from build123d import *

# Parameters (mm, degrees)
F0_R         = 5
F0_R_2       = 1.75
F1_DEPTH     = 5.5
F3_DEPTH     = 3
F4_T4_DEPTH  = 14.8989794856
F4_S5_R      = 5
F4_T6_DEPTH  = 9
F4_T10_DEPTH = 14.8989794856
F4_S11_R     = 5
F4_T12_DEPTH = 9
F5_SIZE      = 0.5


# Not quite as in the source:
# - a fillet or chamfer that OpenCascade refuses, or shapes differently, is made with other operations: its cross-section is extruded or revolved along the edge and cut away or added


with BuildPart() as f1:
    # F0 (on Top) → F1 (new body)
    with BuildSketch(Plane.XY):
        Circle(F0_R)
        Circle(F0_R_2, mode=Mode.SUBTRACT)
    extrude(amount=F1_DEPTH)

    # F2 (on Top) → F3 (join)
    with BuildSketch(Plane.XY):
        with BuildLine():
            Line((0, -5), (4.8989794856, -5))
            ThreePointArc((4.8989794856, -5), (7, 0), (4.8989794856, 5))
            Line((4.8989794856, 5), (0, 5))
            ThreePointArc((0, 5), (5, 0), (0, -5))
        make_face()
    extrude(amount=F3_DEPTH)

    # F4: fillet of radius 2 on 2 edges, made by hand


with BuildPart() as f4_tool2:
    # F4_s3 → F4_t4 (new body)
    with BuildSketch(Plane.YZ.offset(-5)):
        with BuildLine():
            ThreePointArc((-3, 3), (-4.4142135624, 2.4142135624), (-5, 1))
            Line((-5, 1), (-5, 3))
            Line((-5, 3), (-3, 3))
        make_face()
    extrude(amount=F4_T4_DEPTH)

    # F4_s5 → F4_t6 (cut, symmetric)
    with BuildSketch(Plane.XY.offset(2)):
        Circle(F4_S5_R)
    extrude(amount=F4_T6_DEPTH, both=True, mode=Mode.SUBTRACT)


with BuildPart() as f1_1:
    add(f1.part)

    # F4_t1: cut F4_tool2
    add(f4_tool2.part, mode=Mode.SUBTRACT)


with BuildPart() as f4_tool8:
    # F4_s9 → F4_t10 (new body)
    with BuildSketch(Plane.YZ.offset(9.8989794856)):
        with BuildLine():
            ThreePointArc((3, 3), (4.4142135624, 2.4142135624), (5, 1))
            Line((5, 1), (5, 3))
            Line((5, 3), (3, 3))
        make_face()
    extrude(amount=-F4_T10_DEPTH)

    # F4_s11 → F4_t12 (cut, symmetric)
    with BuildSketch(Plane.XY.offset(2)):
        Circle(F4_S11_R)
    extrude(amount=F4_T12_DEPTH, both=True, mode=Mode.SUBTRACT)


with BuildPart() as f1_2:
    add(f1_1.part)

    # F4_t7: cut F4_tool8
    add(f4_tool8.part, mode=Mode.SUBTRACT)

    # F5
    f5_edges = [f1_2.edges().sort_by_distance(p)[0] for p in [
        (-5, 0, 0),
        (2.44949, -5, 0),
        (7, 0, 0),
        (2.44949, 5, 0),
        (-1.75, 0, 0),
    ]]
    chamfer(f5_edges, length=F5_SIZE)


solid = f1_2.part
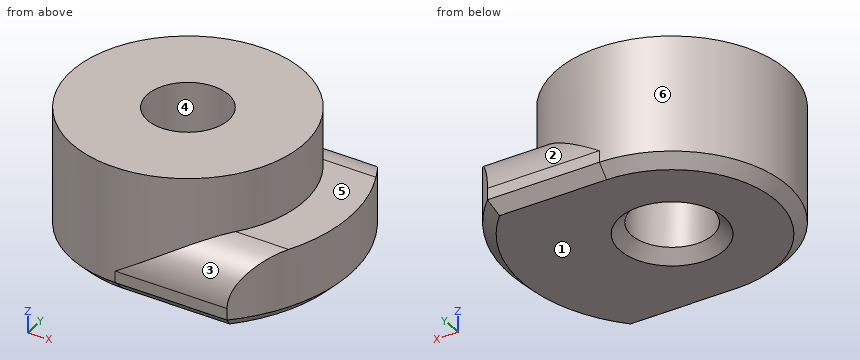
The listing builds one solid part. Answer for the finished solid, in the listing's coordinates (mm). Face numbers are marked on the shaded views. A direction names the side the tool comes from. Coordinates: 2 decimals unless noted, no trailing zeros. Loops run counter-clockwise (first coordinate to the right, second up) from the corner with the lowest first, then second, coordinate; pieces in that order, holes last. Notation, with made-up numbers: (68, 33.25) -> (107, 33.25) arc R10 cw to (107, 47.25) -> close; hole circle Ø7 at (26, 29.5). An arc over 180 degrees is marked (long way). Answer in a Markdown table with one row per item. Add a question column.
1. For the marked faces 1, 2 and 3, determine the directions among +Z, -Z, +X, -X, +Y, -Y from which every point of the face is accessible in a straight line to the end or side of a thin tool.
2. Determine the mould class of the marked faces 4, 5 and 6 for opening direction X: +X half, -X half, draft (parallel to the pull), parting line (faces both ways), or undercut.
3. The part is cut by section A-A, the plane y = 0. Write down the section's boundary in (x, z).
4. The part is cut by section C-C, the plane z = 4. Write down the section's boundary in (x, y), then the cut area to 3 significant figures.
5. Flat-ended cylindrical pins translate along their axes: P1, Ø3.5, axis at x = 6, y = -0.5, coming from the +Z side; P2, Ø1, axis at y = 4, z = 3, coming from the -X side; P3, Ø2, axis at y = -2, z = 4.5, coming from the -X side; P4, Ø3, axis at x = 0, y = 0, coming from the -Z side. Find the tip coordinate at first contact, or state that the pin passes through.
6. Consider line 1 (Y direction, x = 0, z = 1.8); line 2 (X direction, y = -0.75, z = 5.3); line 3 (Z direction, x = 6, y = -0.75). Determine where each line is inside the solid, lowest interval first. Write a range as [from, to].
7. The part is cut by section B-B, the plane z = 1.45. Write down the section's boundary in (x, y).
Answer below:
| question | item | result |
|---|---|---|
| 1 | face 1 | -Z, +X, -X, +Y, -Y |
| 1 | face 2 | +Z, +X, +Y |
| 1 | face 3 | +Z, +X, -Y |
| 2 | face 4 | undercut |
| 2 | face 5 | draft |
| 2 | face 6 | parting line |
| 3 | outline | (-5, 0.5) -> (-4.5, 0) -> (-2.25, 0) -> (-1.75, 0.5) -> (-1.75, 5.5) -> (-5, 5.5) -> close; (1.75, 0.5) -> (2.25, 0) -> (6.5, 0) -> (7, 0.5) -> (7, 3) -> (5, 3) -> (5, 5.5) -> (1.75, 5.5) -> close |
| 4 | outline | circle Ø10 at (0, 0); hole circle Ø3.5 at (0, 0) |
| 4 | area | 68.9 mm2 |
| 5 | P1 | z = 5.5 |
| 5 | P2 | x = -3.57 |
| 5 | P3 | x = -4.9 |
| 5 | P4 | through |
| 6 | line 1 | [-5, -1.75], [1.75, 5] |
| 6 | line 2 | [-4.94, -1.58], [1.58, 4.94] |
| 6 | line 3 | [0, 3] |
| 7 | outline | (0.71, -4.95) -> (4.95, -4.95) arc R7 ccw to (4.95, 4.95) -> (0.71, 4.95) arc R5 ccw (long way) to start; hole circle Ø3.5 at (0, 0) |
